For this review, take the finished solid that the model builds, in its own axes (mm). A direction names the side the tool comes from. Coordinates: 2 decimals unless noted, no trailing zeros. Loops run counter-clockwise (first coordinate to the right, second up) from the corner with the lowest first, then second, coordinate; pieces in that order, holes last. Notation, with made-up numbers: (-3.75, 64) - (35.25, 64) arc R24 cw to (35.25, 82) - close; hole circle Ø10 at (78.5, 75). An arc over 180 degrees is marked (long way). Use one line per item in the form item = value. Start each with the question number.
1. Add section C-C on y = 7.75. Give the boundary of the cut face in (x, z), and give its area (3 significant figures).
2. Add section D-D on z = -7. Give the boundary of the cut face in (x, y), and give its area (3 significant figures).
3. Add section A-A on x = 17.5. Give the boundary of the cut face in (y, z), and give its area (3 significant figures).
4. Add section B-B on z = -2.75. Give the boundary of the cut face in (x, y).
5. Machinability: for faces 1 (the face through (9, 8.382, -4)), 2 (the face through (10, 3.81, -4)), 3 (the face through (0, 2, -2)), which of the approach directions +Z, -Z, +X, -X, +Y, -Y give a long, thin tool a straight path to every point of the face, cutting with its end or side? Answer none if there is none.
6. To check wall thickness, follow probe 1 along Y at (x, z) = (5, -2.5); probe 2 along X at (y, z) = (5.5, -7); probe 3 along Z at (x, y) = (8.5, 4). State the ranges of each line that lie inside material, in increasing order.
7. For pin 1 Ø2 at (x, y) = (16, 5) entering from +Z, flat-tipped, find the tip position at first contact; note if it passes through.
8. Draft analysis for pull direction Y (two halves, no side actions). For faces 4 (the face through (-2.504, 1.526, -3.606)), 5 (the face through (-5.08, 4, -4)), 6 (the face through (10, 4.572, -4)), state which applies: +Y half, -Y half, draft (parallel to the pull), parting line (faces both ways), or undercut.
```python
from build123d import *

# Parameters (mm, degrees)
SKETCH1_W           = 19.05
SKETCH1_H           = 8.382
BOSS_EXTRUDE2_DEPTH = 8.89
SKETCH3_W           = 18.288
SKETCH3_H           = 0.762
CUT_EXTRUDE1_DEPTH  = 7.874
SKETCH4_R           = 2.794
BOSS_EXTRUDE3_DEPTH = 5.08


with BuildPart() as part:
    # Sketch1 → Boss-Extrude2 (new body)
    with BuildSketch(Plane.XY):
        with Locations((9.525, 4.191)):
            Rectangle(SKETCH1_W, SKETCH1_H)
    extrude(amount=-BOSS_EXTRUDE2_DEPTH)

    # Sketch3 → Cut-Extrude1 (cut)
    with BuildSketch(Plane.XY):
        with Locations((9.906, 4.191)):
            Rectangle(SKETCH3_W, SKETCH3_H)
    extrude(amount=-CUT_EXTRUDE1_DEPTH, mode=Mode.SUBTRACT)

    # Sketch4 → Boss-Extrude3 (add)
    with BuildSketch(Plane.ZY):
        with Locations(Location((-4.445, 4.191, 0), (0, 0, 270))):
            Circle(SKETCH4_R)
    extrude(amount=BOSS_EXTRUDE3_DEPTH)


solid = part.part
```
Conclusion:
q1.outline = (0, -8.89) - (19.05, -8.89) - (19.05, 0) - (0, 0) - close
q1.area = 169 mm^2
q2.outline = (-5.08, 3.06) - (0, 3.06) - (0, 0) - (19.05, 0) - (19.05, 3.81) - (0.76, 3.81) - (0.76, 4.57) - (19.05, 4.57) - (19.05, 8.38) - (0, 8.38) - (0, 5.32) - (-5.08, 5.32) - close
q2.area = 157 mm^2
q3.outline = (0, -8.89) - (8.38, -8.89) - (8.38, 0) - (4.57, 0) - (4.57, -7.87) - (3.81, -7.87) - (3.81, 0) - (0, 0) - close
q3.area = 68.5 mm^2
q4.outline = (-5.08, 1.97) - (0, 1.97) - (0, 0) - (19.05, 0) - (19.05, 3.81) - (0.76, 3.81) - (0.76, 4.57) - (19.05, 4.57) - (19.05, 8.38) - (0, 8.38) - (0, 6.41) - (-5.08, 6.41) - close
q5.face_1 = +Z, -Z, +X, -X, +Y
q5.face_2 = +Z, +X
q5.face_3 = -X
q6.probe_1 = 0 to 3.81, 4.57 to 8.38
q6.probe_2 = 0 to 19.05
q6.probe_3 = -8.89 to -7.87
q7.pin_1 = 0
q8.face_4 = parting line
q8.face_5 = draft
q8.face_6 = undercut
